Design review of the part built by this model. Coordinates are the model's own, in mm. Face numbers are marked on the shaded views. A direction names the side the tool comes from. Coordinates: 2 decimals unless noted, no trailing zeros. Loops run counter-clockwise (first coordinate to the right, second up) from the corner with the lowest first, then second, coordinate; pieces in that order, holes last. Notation, with made-up numbers: (-37, 85) -> (-1, 85) arc R25 cw to (-1, 113) -> close; hole circle Ø10 at (-33, 48.25). An arc over 180 degrees is marked (long way). Use a Markdown table: item, result. Add a question column.
Q1. For probe 1 along Z at (x, y) = (-113, 32); probe 2 along X at (y, z) = (31, 82); probe 3 along X at (y, z) = (5.5, 0), list the stretches that pass through material, from the lowest coordinate up.
Q2. Take a section at C-C on x = -28. Write out the cut boundary in (y, z).
Q3. For the marked faces 1 and 2, list the 3-axis set-ups (+Z, -Z, +X, -X, +Y, -Y) from which the entire face can be reached by the end or side of a thin tool; tool diameter is ignored.
Q4. Take a section at A-A on z = 0. Write out the cut boundary in (x, y).
Q5. Take a section at B-B on y = 22. Write out the cut boundary in (x, z), plus the area to 3 significant figures.
Q6. Clearance check with flat-ended pins moving along their axes: pin 1 Ø2 at (x, z) = (115, 2.5) entering from +Y; pin 2 Ø17.5 at (x, z) = (-64.229, 0) entering from +Y (1 decimal). State where each tip first meets the part, or that it passes through.
Q7. Draft analysis for pull direction Z (two halves, no side actions). For the marked faces 3, 4 and 5, state which applies: pulls with the +Z half, pulls with the -Z half, needs draft (parallel to the pull), parting line crosses it, or undercut.
Q8. Take a section at D-D on z = 49.5. Write out the cut boundary in (x, y), plus the area to 3 significant figures.
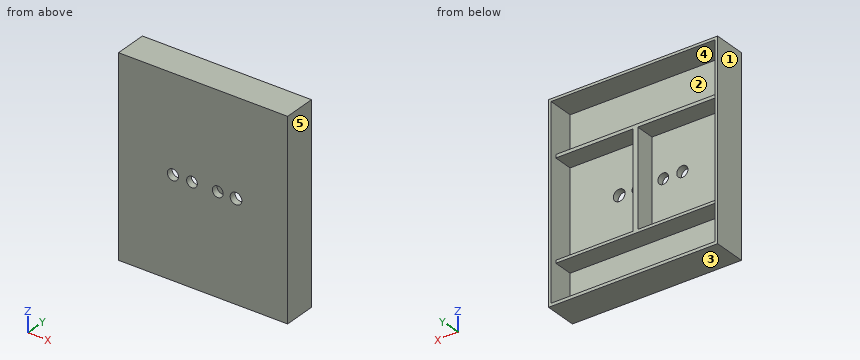
Autodesk Inventor part; units mm, degrees
ref_plane "YZ Plane" through (0, 0, 0) normal (1, 0, 0) x (0, 1, 0)
ref_plane "XZ Plane" through (0, 0, 0) normal (0, 1, 0) x (-1, 0, 0)
ref_plane "XY Plane" through (0, 0, 0) normal (0, 0, 1) x (1, 0, 0)
sketch "Sketch2" plane through (0, 0, 0) normal (0, 1, 0) x (-1, 0, 0)
  line L0 (170.5606, 186.8878) -> (-160.1389, 186.8878)
  line L1 (-160.1389, 186.8878) -> (-160.1389, -194.6885)
  line L2 (-160.1389, -194.6885) -> (170.5606, -194.6885)
  line L3 (170.5606, -194.6885) -> (170.5606, 186.8878)
extrude "Extrusion1" add sketch "Sketch2" along normal blind 12.7
sketch "Sketch4" plane through (0, 12.7, 0) normal (0, 1, 0) x (1, 0, 0)
  line L0 (-170.5606, -186.8878) -> (160.1389, -186.8878)
  line L1 (160.1389, -186.8878) -> (160.1389, 194.6885)
  line L2 (-170.5606, -186.8878) -> (160.1389, -186.8878)
  line L3 (160.1389, -186.8878) -> (160.1389, 194.6885)
  line L4 (160.1389, 194.6885) -> (-170.5606, 194.6885)
  line L5 (-170.5606, 194.6885) -> (-170.5606, -186.8878)
  point P0 (0, 0)
extrude "Extrusion2" add sketch "Sketch4" along normal blind 50.8
sketch "Sketch5" plane through (0, 63.5, 0) normal (0, 1, 0) x (1, 0, 0)
  line L0 (-165.3089, -181.8398) -> (155.2723, -181.8398)
  line L1 (155.2723, -181.8398) -> (155.2723, 188.9245)
  line L2 (155.2723, 188.9245) -> (-165.3089, 188.9245)
  line L3 (-165.3089, 188.9245) -> (-165.3089, -181.8398)
  point P0 (0, 0)
extrude "Extrusion3" cut sketch "Sketch5" against normal blind 50.8
sketch "Sketch9" plane through (0, 12.7, 0) normal (0, 1, 0) x (1, 0, 0)
  line L0 (-165.3089, -181.8398) -> (-165.3089, 188.9245)
  line L1 (155.2723, 188.9245) -> (155.2723, -181.8398)
  line L2 (-165.3089, 109.1943) -> (155.2723, 109.1943)
  line L3 (155.2723, 109.1943) -> (155.2723, 103.846)
  line L4 (155.2723, 103.846) -> (-165.3089, 103.846)
  line L5 (-165.3089, 103.846) -> (-165.3089, 109.1943)
  line L6 (-165.3089, -90.4753) -> (155.2723, -90.4753)
  line L7 (155.2723, -90.4753) -> (155.2723, -84.2356)
  line L8 (155.2723, -84.2356) -> (-165.3089, -84.2356)
  line L9 (-165.3089, -84.2356) -> (-165.3089, -90.4753)
  line L10 (-5.0183, 103.846) -> (4.0112, 103.846)
  line L11 (4.0112, 103.846) -> (4.0112, -84.2356)
  line L12 (4.0112, -84.2356) -> (-5.0183, -84.2356)
  line L13 (-5.0183, -84.2356) -> (-5.0183, 103.846)
  point P0 (0, 0)
extrude "Extrusion6" add sketch "Sketch9" along normal blind 38.1 contours L0 L8 L1 L6 | L0 L2 L1 L4 | L13 L4 L11 L8
sketch "Sketch16" plane through (0, 12.7, 0) normal (0, 1, 0) x (1, 0, 0)
  circle A0 centre (23.4848, 0) radius 10.6311
  circle A1 centre (-26.8974, 0) radius 10.5141
  circle A2 centre (59.1623, 0) radius 11.4331
  circle A3 centre (-64.229, 0) radius 10.9108
  point P0 (0, 0)
extrude "Extrusion10" cut sketch "Sketch16" against normal blind 25.4
properties part number "Base no cutouts.stl"
Answer list:
| question | item | result |
|---|---|---|
| 1 | probe 1 | -194.69 to -188.92, -109.19 to -103.85, 84.24 to 90.48, 181.84 to 186.89 |
| 1 | probe 2 | -170.56 to -165.31, -5.02 to 4.01, 155.27 to 160.14 |
| 1 | probe 3 | -170.56 to -75.14, -53.32 to -37.41, -16.38 to 12.85, 34.12 to 47.73, 70.6 to 160.14 |
| 2 | outline | (0, -194.69) -> (63.5, -194.69) -> (63.5, -188.92) -> (12.7, -188.92) -> (12.7, -109.19) -> (50.8, -109.19) -> (50.8, -103.85) -> (12.7, -103.85) -> (12.7, -10.46) -> (0, -10.46) -> close; (0, 10.46) -> (12.7, 10.46) -> (12.7, 84.24) -> (50.8, 84.24) -> (50.8, 90.48) -> (12.7, 90.48) -> (12.7, 181.84) -> (63.5, 181.84) -> (63.5, 186.89) -> (0, 186.89) -> close |
| 3 | face 1 | +Z, -Z, -X, +Y, -Y |
| 3 | face 2 | +Y |
| 4 | outline | (-170.56, 0) -> (-75.14, 0) -> (-75.14, 12.7) -> (-165.31, 12.7) -> (-165.31, 63.5) -> (-170.56, 63.5) -> close; (-53.32, 0) -> (-37.41, 0) -> (-37.41, 12.7) -> (-53.32, 12.7) -> close; (-16.38, 0) -> (12.85, 0) -> (12.85, 12.7) -> (4.01, 12.7) -> (4.01, 50.8) -> (-5.02, 50.8) -> (-5.02, 12.7) -> (-16.38, 12.7) -> close; (34.12, 0) -> (47.73, 0) -> (47.73, 12.7) -> (34.12, 12.7) -> close; (70.6, 0) -> (160.14, 0) -> (160.14, 63.5) -> (155.27, 63.5) -> (155.27, 12.7) -> (70.6, 12.7) -> close |
| 5 | outline | (-170.56, -194.69) -> (160.14, -194.69) -> (160.14, 186.89) -> (-170.56, 186.89) -> close; hole (-165.31, -188.92) -> (155.27, -188.92) -> (155.27, -109.19) -> (-165.31, -109.19) -> close; hole (-165.31, -103.85) -> (-5.02, -103.85) -> (-5.02, 84.24) -> (-165.31, 84.24) -> close; hole (-165.31, 90.48) -> (155.27, 90.48) -> (155.27, 181.84) -> (-165.31, 181.84) -> close; hole (4.01, -103.85) -> (155.27, -103.85) -> (155.27, 84.24) -> (4.01, 84.24) -> close |
| 5 | area | 12,700 mm² |
| 6 | pin 1 | y = 12.7 |
| 6 | pin 2 | through |
| 7 | face 3 | pulls with the -Z half |
| 7 | face 4 | undercut |
| 7 | face 5 | needs draft |
| 8 | outline | (-170.56, 0) -> (160.14, 0) -> (160.14, 63.5) -> (155.27, 63.5) -> (155.27, 12.7) -> (4.01, 12.7) -> (4.01, 50.8) -> (-5.02, 50.8) -> (-5.02, 12.7) -> (-165.31, 12.7) -> (-165.31, 63.5) -> (-170.56, 63.5) -> close |
| 8 | area | 5,060 mm² |
